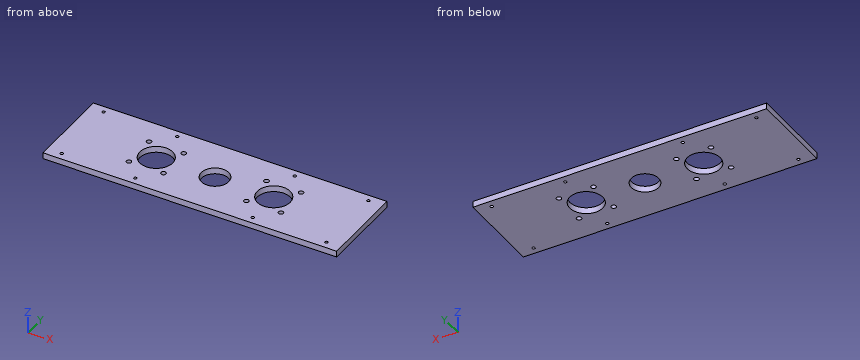
```python
from build123d import *

# Parameters (mm, degrees)
SKETCH1_W           = 304.8
SKETCH1_H           = 89.8
SKETCH1_R           = 14.2875
SKETCH1_R_2         = 2.54
SKETCH1_R_3         = 17.145
BOSS_EXTRUDE1_DEPTH = 6.35
SKETCH2_R           = 1.55
CUT_EXTRUDE1_DEPTH  = 10


with BuildPart() as part:
    # Sketch1 → Boss-Extrude1 (new body)
    with BuildSketch(Plane.XY):
        with Locations((152.4, 44.9)):
            Rectangle(SKETCH1_W, SKETCH1_H)
        with Locations((152.4, 44.9)):
            Circle(SKETCH1_R, mode=Mode.SUBTRACT)
        with Locations((109.401585406, 62.859439014)):
            Circle(SKETCH1_R_2, mode=Mode.SUBTRACT)
        with Locations((109.399439014, 26.938414594)):
            Circle(SKETCH1_R_2, mode=Mode.SUBTRACT)
        with Locations((73.478414594, 26.940560986)):
            Circle(SKETCH1_R_2, mode=Mode.SUBTRACT)
        with Locations((73.480560986, 62.861585406)):
            Circle(SKETCH1_R_2, mode=Mode.SUBTRACT)
        with Locations((91.44, 44.9)):
            Circle(SKETCH1_R_3, mode=Mode.SUBTRACT)
        with Locations((195.400560986, 62.861585406)):
            Circle(SKETCH1_R_2, mode=Mode.SUBTRACT)
        with Locations((231.321585406, 62.859439014)):
            Circle(SKETCH1_R_2, mode=Mode.SUBTRACT)
        with Locations((231.319439014, 26.938414594)):
            Circle(SKETCH1_R_2, mode=Mode.SUBTRACT)
        with Locations((195.398414594, 26.940560986)):
            Circle(SKETCH1_R_2, mode=Mode.SUBTRACT)
        with Locations((213.36, 44.9)):
            Circle(SKETCH1_R_3, mode=Mode.SUBTRACT)
    extrude(amount=BOSS_EXTRUDE1_DEPTH)

    # Sketch2 → Cut-Extrude1 (cut)
    with BuildSketch(Plane(origin=(0, 0, 0), x_dir=(-1, 0, 0), z_dir=(0, 0, -1))):
        with Locations((-289.8, 82.3)):
            Circle(SKETCH2_R)
        with Locations((-213.36, 82.3)):
            Circle(SKETCH2_R)
        with Locations((-91.44, 82.3)):
            Circle(SKETCH2_R)
        with Locations((-15, 82.3)):
            Circle(SKETCH2_R)
        with Locations((-15, 7.5)):
            Circle(SKETCH2_R)
        with Locations((-91.44, 7.5)):
            Circle(SKETCH2_R)
        with Locations((-213.36, 7.5)):
            Circle(SKETCH2_R)
        with Locations((-289.8, 7.5)):
            Circle(SKETCH2_R)
    extrude(amount=-CUT_EXTRUDE1_DEPTH, mode=Mode.SUBTRACT)


solid = part.part
```
Design review of the part built by this model. Coordinates are the model's own, in mm. Coordinates: 2 decimals unless noted, no trailing zeros. Write each loop counter-clockwise with the first axis right and the second up, starting at its lowest first coordinate (ties: lowest second). Pieces come first, ordered by that corner, then holes.
1) Add section A-A (y = 44.9). State how many separate pieces and enclosed holes the cut face has, plus the area to 3 significant figures.
2) Insertion check: pin 1 (1.9 mm diameter, centred on x = 289.8, y = 82.3, fed in from +Z). The pin has a flat end and moves straight along its axis. Give the tip position at first contact, or say it passes through.
3) To check wall thickness, follow L1, parallel to Y at x = 91.44, z = 3.5 (3 decimals); L2, parallel to Y at x = 15, z = 2; L3, parallel to X at y = 82.3, z = 4.25. State the ranges of each line that lie inside material, in increasing order.
4) Add section B-B (x = 152.4). Write out the cut boundary in (y, z), plus the area to 3 significant figures.
Check result:
1. separate pieces: 4
1. enclosed holes: 0
1. area: 1,320 mm2
2. pin 1: passes through
3. L1: y = 0 to 5.95, 9.05 to 27.755, 62.045 to 80.75, 83.85 to 89.8
3. L2: y = 0 to 5.95, 9.05 to 80.75, 83.85 to 89.8
3. L3: x = 0 to 13.45, 16.55 to 89.89, 92.99 to 211.81, 214.91 to 288.25, 291.35 to 304.8
4. outline: (0, 0) - (30.61, 0) - (30.61, 6.35) - (0, 6.35) - close; (59.19, 0) - (89.8, 0) - (89.8, 6.35) - (59.19, 6.35) - close
4. area: 389 mm2
